The model under review builds one solid part; all positions refer to its coordinate system, in mm. A direction names the side the tool comes from. Round coordinates to 2 decimals unless told otherwise and drop trailing zeros. Loops run counter-clockwise (first coordinate to the right, second up) from the corner with the lowest first, then second, coordinate; pieces in that order, holes last. Notation, with made-up numbers: (48, 10.25) -> (77, 10.25) arc R17 cw to (77, 36.25) -> close; hole circle Ø10 at (84, -10). An arc over 180 degrees is marked (long way). Write each question's results on one line, items separated by ' | '. Start each with the question number.
Item 1: We need section D-D (z = -7.25). Give the boundary of the cut face in (x, y), and give its area (3 significant figures).
Item 2: Mouldability with a two-part tool opening along Z and no side actions: class faces 1 (the flat face through (-2, -2, 4)), 2 (the cylindrical face through (-3.905, 2.817, -0.867)), 3 (the cylindrical face through (2.703, -0.986, 8.584)) as pulls with the +Z half, pulls with the -Z half, needs draft (parallel to the pull), parting line crosses it, or undercut.
Item 3: Tool access review of faces 4 (the flat face through (-6, 0, 0)), 5 (the flat face through (-4, 7.5, 2)): name each direction out of +Z, -Z, +X, -X, +Y, -Y from which nothing blocks a thin tool from reaching the whole face with its end or side.
Item 4: Clearance check with flat-ended pins moving along their axes: pin 1 Ø0.5 at (y, z) = (4, -5.5) entering from +X; pin 2 Ø2 at (x, y) = (3.5, 3) entering from +Z; pin 3 Ø2 at (y, z) = (4, -6) entering from -X. State where each tip first meets the part, or that it passes through.
Item 5: We need section B-B (x = 0). Give the boundary of the cut face in (y, z), and give its area (3 significant figures).
Item 6: We need section C-C (x = 7). Give the boundary of the cut face in (y, z), and give its area (3 significant figures).
Item 7: For L1, parallel to X at y = 4.25, z = 0; L2, parallel to Z at x = 2.75, y = 5; L3, parallel to Z at x = 1.25, y = 4.5, list the stretches that pass through material, from the lowest coordinate up. Write a range as from..to.
Item 8: We need section A-A (z = 0). Give the boundary of the cut face in (x, y).
from build123d import *

# Parameters (mm, degrees)
SKETCH1_R           = 5.25
BOSS_EXTRUDE1_DEPTH = 7.5
SKETCH2_W           = 6
SKETCH2_H           = 0.75
SKETCH2_W_2         = 0.75
SKETCH2_H_2         = 6
BOSS_EXTRUDE2_DEPTH = 7.5
SKETCH5_W           = 10
SKETCH5_H           = 10
SKETCH6_R           = 9
BOSS_EXTRUDE3_DEPTH = 2
SKETCH7_R           = 4
CUT_EXTRUDE2_DEPTH  = 16.882380174


with BuildPart() as part:
    # Sketch1 → Boss-Extrude1 (new body)
    with BuildSketch(Plane(origin=(0, 0, 0), x_dir=(1, 0, 0), z_dir=(0, 1, 0))):
        with Locations(Location((0, 0, 0), (0, 0, 270))):
            Circle(SKETCH1_R)
    extrude(amount=BOSS_EXTRUDE1_DEPTH)

    # Sketch2 → Boss-Extrude2 (add)
    with BuildSketch(Plane.XZ):
        with Locations((8, 0)):
            Rectangle(SKETCH2_W, SKETCH2_H)
        Polygon((10.528126947, -3.209231681), (4.73257199, -1.65631741), (4.926686273, -0.931873041), (10.722241231, -2.484787311), align=None)
        Polygon((9.338779442, -5.824759526), (4.142627019, -2.824759526), (4.517627019, -2.175240474), (9.713779442, -5.175240474), align=None)
        Polygon((7.51300955, -8.043339636), (3.270368863, -3.800698949), (3.800698949, -3.270368863), (8.043339636, -7.51300955), align=None)
        Polygon((5.175240474, -9.713779442), (2.175240474, -4.517627019), (2.824759526, -4.142627019), (5.824759526, -9.338779442), align=None)
        Polygon((2.484787311, -10.722241231), (0.931873041, -4.926686273), (1.65631741, -4.73257199), (3.209231681, -10.528126947), align=None)
        with Locations((0, -8)):
            Rectangle(SKETCH2_W_2, SKETCH2_H_2)
        Polygon((-3.209231681, -10.528126947), (-1.65631741, -4.73257199), (-0.931873041, -4.926686273), (-2.484787311, -10.722241231), align=None)
        Polygon((-5.824759526, -9.338779442), (-2.824759526, -4.142627019), (-2.175240474, -4.517627019), (-5.175240474, -9.713779442), align=None)
        Polygon((-8.043339636, -7.51300955), (-3.800698949, -3.270368863), (-3.270368863, -3.800698949), (-7.51300955, -8.043339636), align=None)
        Polygon((-9.713779442, -5.175240474), (-4.517627019, -2.175240474), (-4.142627019, -2.824759526), (-9.338779442, -5.824759526), align=None)
        Polygon((-10.722241231, -2.484787311), (-4.926686273, -0.931873041), (-4.73257199, -1.65631741), (-10.528126947, -3.209231681), align=None)
        with Locations((-8, 0)):
            Rectangle(SKETCH2_W, SKETCH2_H)
        Polygon((-10.528126947, 3.209231681), (-4.73257199, 1.65631741), (-4.926686273, 0.931873041), (-10.722241231, 2.484787311), align=None)
        Polygon((-9.338779442, 5.824759526), (-4.142627019, 2.824759526), (-4.517627019, 2.175240474), (-9.713779442, 5.175240474), align=None)
        Polygon((-7.51300955, 8.043339636), (-3.270368863, 3.800698949), (-3.800698949, 3.270368863), (-8.043339636, 7.51300955), align=None)
        Polygon((-5.175240474, 9.713779442), (-2.175240474, 4.517627019), (-2.824759526, 4.142627019), (-5.824759526, 9.338779442), align=None)
        Polygon((-2.484787311, 10.722241231), (-0.931873041, 4.926686273), (-1.65631741, 4.73257199), (-3.209231681, 10.528126947), align=None)
        with Locations((0, 8)):
            Rectangle(SKETCH2_W_2, SKETCH2_H_2)
        Polygon((3.209231681, 10.528126947), (1.65631741, 4.73257199), (0.931873041, 4.926686273), (2.484787311, 10.722241231), align=None)
        Polygon((5.824759526, 9.338779442), (2.824759526, 4.142627019), (2.175240474, 4.517627019), (5.175240474, 9.713779442), align=None)
        Polygon((8.043339636, 7.51300955), (3.800698949, 3.270368863), (3.270368863, 3.800698949), (7.51300955, 8.043339636), align=None)
        Polygon((9.713779442, 5.175240474), (4.517627019, 2.175240474), (4.142627019, 2.824759526), (9.338779442, 5.824759526), align=None)
        Polygon((10.722241231, 2.484787311), (4.926686273, 0.931873041), (4.73257199, 1.65631741), (10.528126947, 3.209231681), align=None)
    extrude(amount=-BOSS_EXTRUDE2_DEPTH)

    # Sketch5 → Cut-Revolve1 (revolve, cut)
    with BuildSketch(Plane(origin=(0, 0, 0), x_dir=(0, 0, -1), z_dir=(1, 0, 0))):
        with Locations((10.7, 4)):
            Rectangle(SKETCH5_W, SKETCH5_H)
    revolve(axis=Axis((0, 0, 0), (0, 1, 0)), mode=Mode.SUBTRACT)

    # Sketch6 → Boss-Extrude3 (add)
    with BuildSketch(Plane(origin=(0, 0, 0), x_dir=(1, 0, 0), z_dir=(0, 1, 0))):
        with Locations(Location((0, 0, 0), (0, 0, 270))):
            Circle(SKETCH6_R)
    extrude(amount=-BOSS_EXTRUDE3_DEPTH)

    # Sketch7 → Cut-Extrude2 (cut, through all)
    with BuildSketch(Plane(origin=(0, 7.5, 0), x_dir=(1, 0, 0), z_dir=(0, 1, 0))):
        with Locations(Location((0, 0, 0), (0, 0, 270))):
            Circle(SKETCH7_R)
    extrude(amount=-CUT_EXTRUDE2_DEPTH, mode=Mode.SUBTRACT)


solid = part.part
Here are the results:
1) outline: (-5.33, -2) -> (5.33, -2) -> (5.33, 0) -> (-5.33, 0) -> close | area: 21.3 mm2
2) face 1: needs draft | face 2: undercut | face 3: parting line crosses it
3) face 4: +Y | face 5: +Z, -Z, +X, -X, +Y
4) pin 1: stops at x = 1.83 | pin 2: stops at z = 5.11 | pin 3: stops at x = -2.74
5) outline: (-2, -9) -> (0, -9) -> (0, -5.7) -> (7.5, -5.7) -> (7.5, -4) -> (-2, -4) -> close; (-2, 4) -> (7.5, 4) -> (7.5, 5.7) -> (0, 5.7) -> (0, 9) -> (-2, 9) -> close | area: 45.5 mm2
6) outline: (-2, -5.66) -> (0, -5.66) -> (0, 5.66) -> (-2, 5.66) -> close | area: 22.6 mm2
7) L1: x = -5.7..-4, 4..5.7 | L2: z = -4.99..-2.9, 2.9..4.99 | L3: z = -5.56..-3.8, 3.8..5.56
8) outline: (-9, -2) -> (-4, -2) -> (-4, 7.5) -> (-5.7, 7.5) -> (-5.7, 0) -> (-9, 0) -> close; (4, -2) -> (9, -2) -> (9, 0) -> (5.7, 0) -> (5.7, 7.5) -> (4, 7.5) -> close
